```python
from build123d import *

# Parameters (mm, degrees)
F0_R     = 250
F2_DEPTH = 500
F1_R     = 250
F1_W     = 200
F1_H     = 200
F3_DEPTH = 1500
F1_W_2   = 959.411026
F1_H_2   = 659
F4_DEPTH = 25
F6_DEPTH = 2000


with BuildPart() as f2:
    # F0 (on Front) → F2 (new body)
    with BuildSketch(Plane.XZ):
        Circle(F0_R)
    extrude(amount=F2_DEPTH)

    # F1 (on face) → F3 (join)
    with BuildSketch(Plane.XZ):
        Circle(F1_R)
        Rectangle(F1_W, F1_H, mode=Mode.SUBTRACT)
        Rectangle(F1_W, F1_H)
    extrude(amount=-F3_DEPTH)

    # F1 (on face) → F4 (cut)
    with BuildSketch(Plane.XZ):
        Rectangle(F1_W_2, F1_H_2)
        Rectangle(F1_W, F1_H, mode=Mode.SUBTRACT)
    extrude(amount=-F4_DEPTH, mode=Mode.SUBTRACT)

    # F5 (on face) → F6 (intersect)
    with BuildSketch(Plane.XZ.offset(500)):
        with BuildLine():
            Line((0, 250), (0, 0))
            Line((0, 0), (21.788936, 249.048675))
            ThreePointArc((21.788936, 249.048675), (10.904847, 249.762055), (0, 250))
        make_face()
    extrude(amount=-F6_DEPTH, mode=Mode.INTERSECT)


solid = f2.part
```
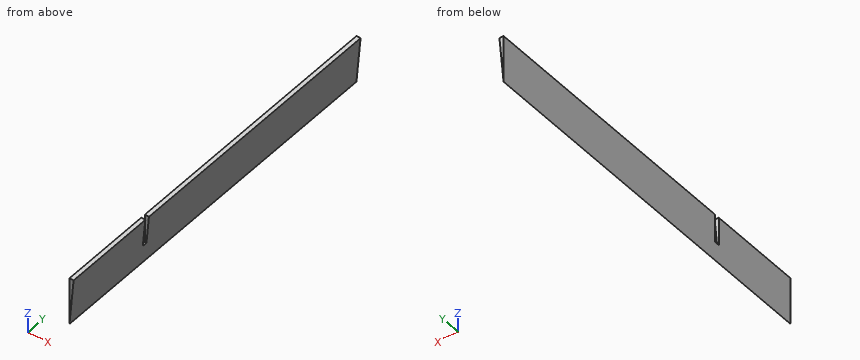
Can you work these out from the model? Positions are in its coordinate system, mm. Round coordinates to 2 decimals unless told otherwise and drop trailing zeros. Loops run counter-clockwise (first coordinate to the right, second up) from the corner with the lowest first, then second, coordinate; pieces in that order, holes last. Notation, with made-up numbers: M 48,51 L 82,51 A13 cw 82,67 Z; hole C 28,-10.5 d10. An arc over 180 degrees is marked long. Answer in a Markdown table with one row per item.
1. If we section it at D-D, the plane z = 65.5: Please give me the cut outline in (x, y).
Established:
| item | result |
|---|---|
| outline | M 0,-500 L 5.73,-500 L 5.73,1500 L 0,1500 Z |
2. If we section it at A-A, the plane z = 180: Please give me the cut outline in (x, y).
Established:
| item | result |
|---|---|
| outline | M 0,-500 L 15.75,-500 L 15.75,0 L 0,0 Z; M 0,25 L 15.75,25 L 15.75,1500 L 0,1500 Z |
3. I'm going to push flat-ended pins straight in: pin 1 Ø7 at (x, y) = (5.5, 10) entering from +Z; pin 2 Ø5 at (y, z) = (786.5, 168.5) entering from +X; pin 3 Ø10 at (y, z) = (-249, 122) entering from +X. Where does each tip first touch, or does it pass through?
Established:
| item | result |
|---|---|
| pin 1 | z = 100 |
| pin 2 | x = 14.96 |
| pin 3 | x = 11.11 |
4. Please list where these lines run through material, in increasing order: line 1 (Y direction, x = 9.5, z = 198); line 2 (X direction, y = 1342, z = 100); line 3 (X direction, y = 14, z = 95.5). Write a range as from..to.
Established:
| item | result |
|---|---|
| line 1 | -500..0, 25..1500 |
| line 2 | 0..8.75 |
| line 3 | 0..8.36 |
5. If we section it at B-B, the plane x = 17.25: Please give me the cut outline in (y, z), plus the area to 3 significant figures.
Established:
| item | result |
|---|---|
| outline | M -500,197.17 L 0,197.17 L 0,249.4 L -500,249.4 Z; M 25,197.17 L 1500,197.17 L 1500,249.4 L 25,249.4 Z |
| area | 103,000 mm² |
6. If we section it at C-C, the plane y = 850: Please give me the cut outline in (x, z).
Established:
| item | result |
|---|---|
| outline | M 0,0 L 21.79,249.05 A250 ccw 0,250 Z |
